Design review of the part built by this model. Coordinates are the model's own, in mm. Face numbers are marked on the shaded views. A direction names the side the tool comes from. Coordinates: 2 decimals unless noted, no trailing zeros. Write each loop counter-clockwise with the first axis right and the second up, starting at its lowest first coordinate (ties: lowest second). Pieces come first, ordered by that corner, then holes. Notation, with made-up numbers: (67.25, -13.5) -> (95.25, -13.5) arc R22 cw to (95.25, 25.5) -> close; hole circle Ø9 at (22, 64). An arc over 180 degrees is marked (long way). Answer in a Markdown table with one row per item. Add a question column.
Item 1: Clearance check with flat-ended pins moving along their axes: P1, Ø5, axis at x = 54.5, z = -65, coming from the -Y side; P2, Ø4, axis at x = 87.5, z = -91, coming from the +Y side. State where each tip first meets the part, or that it passes through.
Item 2: Take a section at B-B, the plane y = 1.4. Write out the cut boundary in (x, z), and give its area (3 significant figures).
Item 3: To check wall thickness, follow line 1 (Y direction, x = 95.5, z = -79); line 2 (X direction, y = 1.2, z = -80); line 3 (X direction, y = 0.8, z = -56.5). State the ranges of each line that lie inside material, in increasing order.
Item 4: Take a section at D-D, the plane z = -66.5. Write out the cut boundary in (x, y).
Item 5: Take a section at C-C, the plane x = 38. Write out the cut boundary in (y, z).
Item 6: Take a section at A-A, the plane z = -120. Write out the cut boundary in (x, y), and give its area (3 significant figures).
Item 7: For the marked faces 1 and 2, list the 3-axis set-ups (+Z, -Z, +X, -X, +Y, -Y) from which the entire face can be reached by the end or side of a thin tool; tool diameter is ignored.
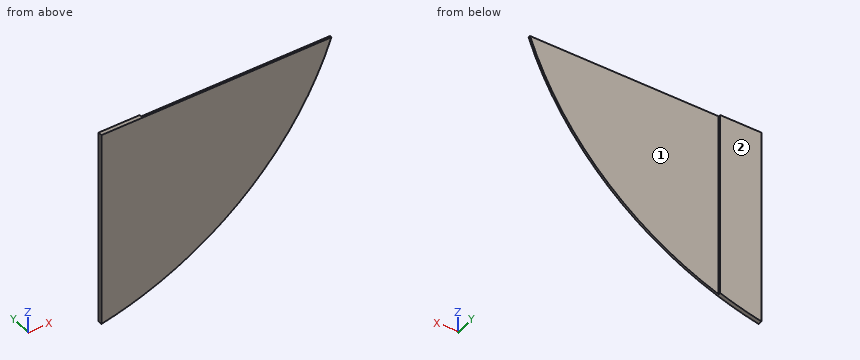
from build123d import *

# Parameters (mm, degrees)
BOSS_EXTRUDE3_DEPTH = 1
BOSS_EXTRUDE4_DEPTH = 1
CUT_EXTRUDE1_DEPTH  = 208.84850252


with BuildPart() as part:
    # Sketch1 → Boss-Extrude3 (new body)
    with BuildSketch(Plane(origin=(0, 0, 0), x_dir=(1, 0, 0), z_dir=(0, 1, 0))):
        with BuildLine():
            Line((50, 141.421356237), (50, 50))
            Line((50, 50), (141.421356237, 50))
            ThreePointArc((141.421356237, 50), (106.066017178, 106.066017178), (50, 141.421356237))
        make_face()
        with BuildLine():
            Line((30, 50), (50, 50))
            Line((50, 50), (50, 141.421356237))
            ThreePointArc((50, 141.421356237), (40.096074055, 144.541706249), (30, 146.969384567))
            Line((30, 146.969384567), (30, 50))
        make_face()
        with BuildLine():
            Line((50, 50), (50, 30))
            Line((50, 30), (146.969384567, 30))
            ThreePointArc((146.969384567, 30), (144.541706249, 40.096074055), (141.421356237, 50))
            Line((141.421356237, 50), (50, 50))
        make_face()
    extrude(amount=BOSS_EXTRUDE3_DEPTH)

    # Sketch2 → Boss-Extrude4 (add)
    with BuildSketch(Plane(origin=(0, 1, 0), x_dir=(-1, 0, 0), z_dir=(0, 1, 0))):
        with BuildLine():
            Line((-50, -50), (-30, -50))
            Line((-30, -50), (-30, -146.969384567))
            ThreePointArc((-30, -146.969384567), (-40.096074055, -144.541706249), (-50, -141.421356237))
            Line((-50, -141.421356237), (-50, -50))
        make_face()
    extrude(amount=BOSS_EXTRUDE4_DEPTH)

    # Sketch3 → Cut-Extrude1 (cut, through all)
    with BuildSketch(Plane(origin=(0, 1, 0), x_dir=(-1, 0, 0), z_dir=(0, 1, 0))):
        with BuildLine():
            Line((-141.421356237, -50), (-50, -50))
            Line((-50, -50), (-50, -30))
            Line((-50, -30), (-146.969384567, -30))
            ThreePointArc((-146.969384567, -30), (-144.541706249, -40.096074055), (-141.421356237, -50))
        make_face()
    extrude(amount=-CUT_EXTRUDE1_DEPTH, mode=Mode.SUBTRACT)


solid = part.part
Answers:
| question | item | result |
|---|---|---|
| 1 | P1 | stops at y = 0 |
| 1 | P2 | stops at y = 1 |
| 2 | outline | (30, -146.97) arc R150 ccw to (50, -141.42) -> (50, -50) -> (30, -50) -> close |
| 2 | area | 1,890 mm^2 |
| 3 | line 1 | y = 0 to 1 |
| 3 | line 2 | x = 30 to 50 |
| 3 | line 3 | x = 30 to 138.95 |
| 4 | outline | (30, 0) -> (134.45, 0) -> (134.45, 1) -> (50, 1) -> (50, 2) -> (30, 2) -> close |
| 5 | outline | (0, -145.11) -> (2, -145.11) -> (2, -50) -> (0, -50) -> close |
| 6 | outline | (30, 0) -> (90, 0) -> (90, 1) -> (50, 1) -> (50, 2) -> (30, 2) -> close |
| 6 | area | 80.0 mm^2 |
| 7 | face 1 | +Z, -Z, +X, +Y |
| 7 | face 2 | +Z, -Z, +X, -X, +Y |
